Model file for the job. Use its own axes, mm. A direction names the side the tool comes from. Round coordinates to 2 decimals unless told otherwise and drop trailing zeros. Write each loop counter-clockwise with the first axis right and the second up, starting at its lowest first coordinate (ties: lowest second). Pieces come first, ordered by that corner, then holes. Notation, with made-up numbers: (-37.5, -13.75) - (-18.5, -13.75) arc R24 cw to (-18.5, 6.25) - close; hole circle Ø10 at (89.25, 30). An arc over 180 degrees is marked (long way). Answer as a JSON object with one key per item and string values. Group by question number.
Autodesk Inventor part; units mm, degrees
ref_plane "YZ Plane" through (0, 0, 0) normal (1, 0, 0) x (0, 1, 0)
ref_plane "XZ Plane" through (0, 0, 0) normal (0, 1, 0) x (-1, 0, 0)
ref_plane "XY Plane" through (0, 0, 0) normal (0, 0, 1) x (1, 0, 0)
sketch "Boceto1" plane through (0, 0, 0) normal (0, 0, 1) x (1, 0, 0)
  line L0 (186.1, 8.9) -> (186.1, -186.1)
  line L1 (-8.9, 8.9) -> (-8.9, -186.1)
  line L2 (186.1, -186.1) -> (-8.9, -186.1)
  line L3 (-8.9, 8.9) -> (186.1, 8.9)
  point P0 (0, 0)
extrude "Extrusión1" add sketch "Boceto1" along normal blind 4.4
sketch "Boceto2" plane through (0, 0, 4.4) normal (0, 0, 1) x (1, 0, 0)
  line L0 (186.1, -186.1) -> (186.1, 8.9)
  line L1 (-8.9, -186.1) -> (186.1, -186.1)
  line L2 (-8.9, 8.9) -> (-8.9, -186.1)
  line L3 (186.1, 8.9) -> (-8.9, 8.9)
  circle A0 centre (88.6021, -88.6021) radius 35
  point P0 (0, 0)
  dimension "d2" = 70
  dimension "d3" = 97.4979
  dimension "d4" = 97.4979
extrude "Extrusión2" add sketch "Boceto2" along normal blind 26.5 contours A0
properties part number "Acrilico_Top"
(1) Slice it at D-D (z = 20.5). Write the cut outline in (x, y).
(2) 3-axis set-ups, long thin cutter, end or side, ignore diameter. For faces 1 (the flat face through (90, -186.1, 2)), 2 (the flat face through (44, -87, 4.4)): which of +Z, -Z, +X, -X, +Y, -Y reach the whole face in a straight line?
(3) Slice it at B-B (y = -84). Write the cut outline in (x, z), then the cut area to 3 significant figures.
(4) Slice it at C-C (x = 127). Write the cut outline in (y, z).
(5) Slice it at A-A (x = 86). Write the cut outline in (y, z), then the cut area to 3 significant figures.
(6) Drill centre lines: line 1 (Z direction, x = 44, y = -7); line 2 (X direction, y = -98, z = 14); line 3 (Y direction, x = 109, z = 17). Where is each one in solid material? Low to high. Write a range as from..to.
(7) Flat gauge pins, fed straight in: pin 1 (4 mm diameter, centred on y = -107.5, z = 19, fed in from +X); pin 2 (1 mm diameter, centred on y = -125.5, z = 15, fed in from -X); pin 3 (3 mm diameter, centred on y = -89, z = 28, fed in from -X); pin 4 (5 mm diameter, centred on x = 82.5, z = 19, fed in from -Y). Where does each tip first touch, or does it go through?
Answer:
{
 "1": {"outline": "circle Ø70 at (88.6, -88.6)"},
 "2": {"face 1": "+Z, -Z, +X, -X, -Y", "face 2": "+Z"},
 "3": {"outline": "(-8.9, 0) - (186.1, 0) - (186.1, 4.4) - (123.3, 4.4) - (123.3, 30.9) - (53.91, 30.9) - (53.91, 4.4) - (-8.9, 4.4) - close", "area": "2,700 mm²"},
 "4": {"outline": "(-186.1, 0) - (8.9, 0) - (8.9, 4.4) - (-186.1, 4.4) - close"},
 "5": {"outline": "(-186.1, 0) - (8.9, 0) - (8.9, 4.4) - (-53.7, 4.4) - (-53.7, 30.9) - (-123.51, 30.9) - (-123.51, 4.4) - (-186.1, 4.4) - close", "area": "2,710 mm²"},
 "6": {"line 1": "0..4.4", "line 2": "54.89..122.32", "line 3": "-117.04..-60.16"},
 "7": {"pin 1": "x = 119.25", "pin 2": "through", "pin 3": "x = 53.6", "pin 4": "y = -123.42"}
}
